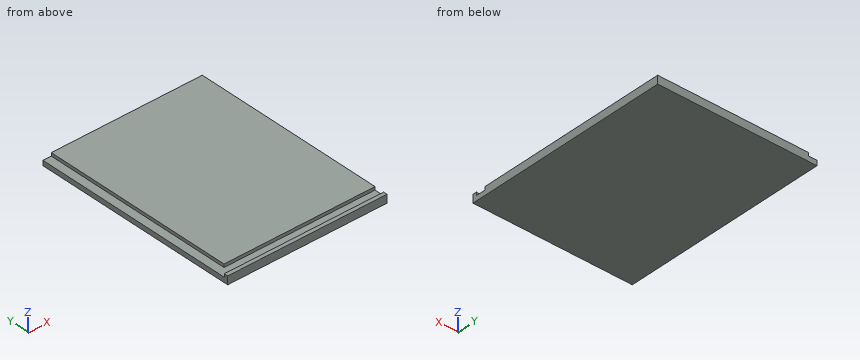
```python
from build123d import *

# Parameters (mm, degrees)
SKETCH006_W     = 250
SKETCH006_H     = 325
PAD005_DEPTH    = 12.7
POCKET001_DEPTH = 5


with BuildPart() as roof:
    # Sketch006 → Pad005 (new body)
    with BuildSketch(Plane.XY):
        with Locations((742.936954, 526.654633)):
            Rectangle(SKETCH006_W, SKETCH006_H)
    extrude(amount=PAD005_DEPTH)

    # Sketch007 (on Face6 of Pad005) → Pocket001 (cut)
    with BuildSketch(Plane.XY.offset(12.7)):
        Polygon((854.936954, 702.879578), (854.936954, 385.154633), (607.793213, 385.154633), (607.793213, 370.154633), (885.780701, 370.154633), (885.780701, 702.879578), align=None)
    extrude(amount=-POCKET001_DEPTH, mode=Mode.SUBTRACT)


with BuildPart() as model_roof_mirrored:
    # Mirror001: instance of Roof
    add(roof.part.mirror(Plane(origin=(875.298889, 692.274536, 0), x_dir=(0, 1, 0), z_dir=(-1, 0, 0))))


solid = model_roof_mirrored.part
```
Geometry: final body of the model. Coordinates: model frame, mm. Round coordinates to 2 decimals unless told otherwise and drop trailing zeros. Write each loop counter-clockwise with the first axis right and the second up, starting at its lowest first coordinate (ties: lowest second). Pieces come first, ordered by that corner, then holes.
Item 1: Section query A-A (z = 10). Return loops of the section in (x, y).
Item 2: Section query B-B (y = 617). Return loops of the section in (x, z), plus the area to 3 significant figures.
Item 3: Material intervals for L1, parallel to Y at x = 1015, z = 8; L2, parallel to X at y = 539.5, z = 12.25, sorted ascending.
Item 4: Section query C-C (x = 1030). Return loops of the section in (y, z), plus the area to 3 significant figures.
Completed:
1. outline: (882.66, 364.15) - (1132.66, 364.15) - (1132.66, 370.15) - (882.66, 370.15) - close; (895.66, 385.15) - (1132.66, 385.15) - (1132.66, 689.15) - (895.66, 689.15) - close
2. outline: (882.66, 0) - (1132.66, 0) - (1132.66, 12.7) - (895.66, 12.7) - (895.66, 7.7) - (882.66, 7.7) - close
2. area: 3,110 mm2
3. L1: y = 364.15 to 370.15, 385.15 to 689.15
3. L2: x = 895.66 to 1132.66
4. outline: (364.15, 0) - (689.15, 0) - (689.15, 12.7) - (385.15, 12.7) - (385.15, 7.7) - (370.15, 7.7) - (370.15, 12.7) - (364.15, 12.7) - close
4. area: 4,050 mm2
